For this review, take the finished solid that the model builds, in its own axes (mm). Face numbers are marked on the shaded views. Coordinates: 2 decimals unless noted, no trailing zeros.
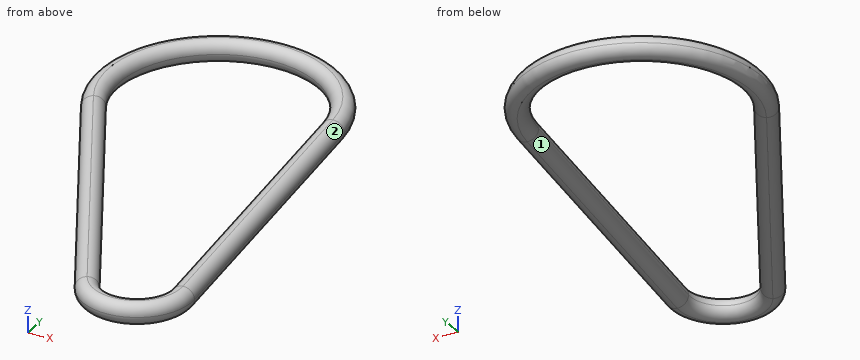
Autodesk Inventor part; units mm, degrees
ref_plane "YZ Plane" through (0, 0, 0) normal (1, 0, 0) x (0, 1, 0)
ref_plane "XZ Plane" through (0, 0, 0) normal (0, 1, 0) x (-1, 0, 0)
ref_plane "XY Plane" through (0, 0, 0) normal (0, 0, 1) x (1, 0, 0)
ref_plane "作業平面1" through (0, 0, 0) normal (0, 0, 1) x (1, 0, 0)
sketch "スケッチ1" plane through (0, 0, 0) normal (0, 0, 1) x (1, 0, 0)
  circle A0 centre (1.4986, -6.7164) radius 2.5
  circle A1 centre (-2.9986, 8.2164) radius 5.5
  line L0 (2.4745, 8.7597) -> (3.9863, -6.4695)
  line L1 (-7.8615, 5.647) -> (-0.7119, -7.8843)
  arc A2 (1.4794, 8.6609) -> (-6.9773, 6.1141) centre (-2.9986, 8.2164) ccw
  line L2 (1.4794, 8.6609) -> (2.9912, -6.5682)
  arc A3 (0.1723, -7.4172) -> (2.9912, -6.5682) centre (1.4986, -6.7164) ccw
  line L3 (-6.9773, 6.1141) -> (0.1723, -7.4172)
  point P0 (0, 0)
  dimension "d0" = 1
  dimension "d1" = 1
extrude "押し出し1" add sketch "スケッチ1" along normal blind 1 contours A0 L3 A3 L2 | A0 L2 A1 L0 | L1 A1 L3 A0 | A1 L2 A2 L3 picked at (3.0117, -5.3596) picked at (-6.3062, 4.4531)
fillet "フィレット1" radius 0.5 16 edges at (-4.5846, 13.4828, 1) (-4.2867, -1.1187, 1) (2.2195, -9.1102, 1) (3.2304, 1.1451, 1) (-4.5846, 13.4828, 0) (-4.2867, -1.1187, 0) (2.2195, -9.1102, 0) (3.2304, 1.1451, 0) (1.9311, -8.1527, 1) (-3.4025, -0.6515, 1) (-4.2962, 12.5253, 1) (2.2353, 1.0464, 1) (1.9311, -8.1527, 0) (-3.4025, -0.6515, 0) (-4.2962, 12.5253, 0) (2.2353, 1.0464, 0)
properties part number "Belt"
Q1. For probe 1 along Y at (x, z) = (-1, 0.45); probe 2 along Y at (x, z) = (-6.5, 0.8); probe 3 along X at (y, z) = (2, 0.75), list the stretches that pass through material, from the lowest coordinate up.
Ans:
probe 1: y = -7.33 to -5.2, 12.25 to 13.34
probe 2: y = 3.28 to 5, 11.2 to 12.33
probe 3: x = -5.86 to -4.88, 2.21 to 3.08
Q2. Clearance check with a flat-ended pin moving along its axis: pin 1 Ø3 at (x, y) = (-2.5, 0.5) entering from +Z. State where the tip first meets the part, or that it passes through.
Ans:
pin 1: stops at z = 0.87
Q3. Draft analysis for pull direction X (two halves, no side actions). For the marked faces 1 and 2, state which applies: +X half, -X half, draft (parallel to the pull), parting line (faces both ways), or undercut.
Ans:
face 1: undercut
face 2: +X half
